Model file for the job. Use its own axes, mm. Coordinates: 2 decimals unless noted, no trailing zeros. Write each loop counter-clockwise with the first axis right and the second up, starting at its lowest first coordinate (ties: lowest second). Pieces come first, ordered by that corner, then holes. Notation, with made-up numbers: (-31.75, 86) - (-8.75, 86) arc R23 cw to (-8.75, 121) - close; hole circle Ø8 at (3.5, 52). An arc over 180 degrees is marked (long way). Put each result on its own line as item: value. Start each with the question number.
1. Drill centre lines: L1, parallel to Z at x = 47, y = -0.35; L2, parallel to Z at x = 45, y = -0.75; L3, parallel to Z at x = -49, y = -0.1. Where is each one in solid material? Low to high. Write a range as from..to.
2. Drop flat-ended pins along their axis: P1, Ø0.5, axis at y = -0.5, z = -14, coming from the -X side; P2, Ø5, axis at x = 40, z = -2.5, coming from the -Y side; P3, Ø0.5, axis at y = -0.5, z = -10.5, coming from the +X side. Give the stop position or say it passes through.
3. Saw through at A-A, the plane x = -18.5. Write the cut outline in (y, z), plus the area to 3 significant figures.
4. Saw through at C-C, the plane x = 20. Write the cut outline in (y, z).
5. Saw through at B-B, the plane y = -0.75. Give the number of separate pieces and of enclosed holes in the cut face, plus the area to 3 significant figures.
```python
from build123d import *

# Parameters (mm, degrees)
F0_W     = 0.1
F0_H     = 0.5
F0_W_2   = 4.5762195215
F0_H_2   = 0.1
F0_W_3   = 15
F0_H_3   = 7
F0_W_4   = 4
F0_W_5   = 5.7000000263
F0_W_6   = 6
F0_H_4   = 8
F0_W_7   = 2.1349615479
F0_W_8   = 5.4599995956
F0_H_5   = 1.8540623203
F0_H_6   = 1.1455476638
F0_W_9   = 7.5237791166
F0_W_10  = 2
F0_W_11  = 3.1167556109
F0_H_7   = 0.894062461
F0_W_12  = 8
F0_W_13  = 1.8985043958
F0_W_14  = 5.535091728
F0_W_15  = 2.1720023397
F0_W_16  = 5
F0_H_8   = 5
F0_W_17  = 9
F0_H_9   = 6
F0_W_18  = 3.3521689058
F1_DEPTH = 1


with BuildPart() as f1:
    # F0 (on Front) → F1 (new body)
    with BuildSketch(Plane.XZ):
        Polygon((-0.7164276307, -4), (-1.7164276307, -4), (-1.7164276307, 2.0474093835), (21.9873721178, 2.0474093835), (21.9873721178, -2.9525906165), (1.9873721178, -2.9525906165), (0.2835723693, -4), (-0.6164276307, -4), (-0.6164276307, -4.5), (0.4249689693, -4.5), (2.1287687179, -3.4525906165), (22.4873721178, -3.4525906165), (22.4873721178, -0.1), (22.4873721178, 0), (22.4873721178, 2.5474093835), (-2.2164276307, 2.5474093835), (-2.2164276307, 0), (-2.2164276307, -0.1), (-2.2164276307, -4.5), (-0.7164276307, -4.5), align=None)
        with Locations((-0.6664276307, -4.25)):
            Rectangle(F0_W, F0_H)
        with BuildLine():
            Line((-0.6164276307, -4.5), (-0.7164276307, -4.5))
            Line((-0.7164276307, -4.5), (-0.7164276307, -13.3747674979))
            ThreePointArc((-0.7164276307, -13.3747674979), (-0.6663757902, -13.3759068091), (-0.6164276307, -13.3793223828))
            Line((-0.6164276307, -13.3793223828), (-0.6164276307, -4.5))
        make_face()
        with BuildLine():
            ThreePointArc((-0.6164276307, -13.3793223828), (-0.6663757902, -13.3759068091), (-0.7164276307, -13.3747674979))
            ThreePointArc((-0.7164276307, -13.3747674979), (-1.8164276307, -14.4747674979), (-0.7164276307, -15.5747674979))
            Line((-0.7164276307, -15.5747674979), (-0.7164276307, -15.4747674979))
            ThreePointArc((-0.7164276307, -15.4747674979), (-1.4235344119, -13.7676607167), (0.2835723693, -14.4747674979))
            ThreePointArc((0.2835723693, -14.4747674979), (0.025192218, -15.1455878911), (-0.6164276307, -15.469754935))
            Line((-0.6164276307, -15.469754935), (-0.6164276307, -15.5702126129))
            ThreePointArc((-0.6164276307, -15.5702126129), (0.0559267082, -15.2580099731), (0.3775103589, -14.5900917138))
            ThreePointArc((0.3775103589, -14.5900917138), (0.3816245836, -14.5401994065), (0.3834645069, -14.4901715758))
            ThreePointArc((0.3834645069, -14.4901715758), (0.3835454033, -14.4824697256), (0.3835723693, -14.4747674979))
            ThreePointArc((0.3835723693, -14.4747674979), (0.0959762097, -13.7331476491), (-0.6164276307, -13.3793223828))
        make_face()
        with BuildLine():
            Line((-0.7164276307, -15.4747674979), (-0.7164276307, -15.5747674979))
            ThreePointArc((-0.7164276307, -15.5747674979), (-0.6663757902, -15.5736281866), (-0.6164276307, -15.5702126129))
            Line((-0.6164276307, -15.5702126129), (-0.6164276307, -15.469754935))
            ThreePointArc((-0.6164276307, -15.469754935), (-0.6663648557, -15.473513571), (-0.7164276307, -15.4747674979))
        make_face()
        with BuildLine():
            ThreePointArc((-0.6164276307, -15.5702126129), (-0.6663757902, -15.5736281866), (-0.7164276307, -15.5747674979))
            Line((-0.7164276307, -15.5747674979), (-0.7164276307, -16.196783632))
            Line((-0.7164276307, -16.196783632), (-0.6164276307, -16.196783632))
            Line((-0.6164276307, -16.196783632), (-0.6164276307, -15.5702126129))
        make_face()
        with Locations((-4.5045373915, -0.05)):
            Rectangle(F0_W_2, F0_H_2)
        Polygon((-6.7926471522, -5.3350963127), (-6.7926471522, -0.1), (-6.7926471522, 0), (-6.7926471522, 2.6649036873), (-22.7926471522, 2.6649036873), (-22.7926471522, 0), (-22.7926471522, -0.1), (-22.7926471522, -5.3350963127), align=None)
        with Locations((-14.7926471522, -1.3350963127)):
            Rectangle(F0_W_3, F0_H_3, mode=Mode.SUBTRACT)
        with BuildLine():
            Line((44.9668482701, -15.1770115764), (0.3834645069, -14.4901715758))
            ThreePointArc((0.3834645069, -14.4901715758), (0.3816245836, -14.5401994065), (0.3775103589, -14.5900917138))
            Line((0.3775103589, -14.5900917138), (44.9668482701, -15.2770234426))
            Line((44.9668482701, -15.2770234426), (45.0668482701, -15.2785640165))
            Line((45.0668482701, -15.2785640165), (45.0668482701, -15.1785521504))
            Line((45.0668482701, -15.1785521504), (45.0668482701, -13.2785640165))
            Line((45.0668482701, -13.2785640165), (44.9668482701, -13.2785640165))
            Line((44.9668482701, -13.2785640165), (44.9668482701, -15.1770115764))
        make_face()
        with Locations((24.4873721178, -0.05)):
            Rectangle(F0_W_4, F0_H_2)
        Polygon((26.4873721178, 0), (26.4873721178, -0.1), (26.4873721178, -2.6669805495), (29.4873721178, -3.0982994409), (29.5873721178, -3.1126767373), (32.4873721178, -3.5296183324), (32.4873721178, 0), (32.4873721178, 0.1), (32.4873721178, 2.5474093835), (26.4873721178, 2.5474093835), (26.4873721178, 0.0474093835), align=None)
        Polygon((26.9873721178, -2.2337257974), (26.9873721178, 0.0474093835), (26.9873721178, 2.0474093835), (31.9873721178, 2.0474093835), (31.9873721178, -2.9525906165), (29.5873721178, -2.6075355033), align=None, mode=Mode.SUBTRACT)
        Polygon((44.0542930675, -13.2785640165), (44.9668482701, -13.2785640165), (45.0668482701, -13.2785640165), (46.0794034727, -13.2785640165), (46.5562570157, -12.0984218523), (52.1539116397, -12.0984218523), (52.1539116397, -9.4984218523), (44.0542930675, -9.4984218523), (44.0542930675, -10.1705333218), (44.0542930675, -10.2705333218), align=None)
        Polygon((51.8539116397, -11.7984218523), (46.3539116397, -11.7984218523), (45.8770580967, -12.9785640165), (44.3542930675, -12.9785640165), (44.3542930675, -9.7984218523), (51.8539116397, -9.7984218523), align=None, mode=Mode.SUBTRACT)
        with Locations((-25.6426471653, -0.05)):
            Rectangle(F0_W_5, F0_H_2)
        Polygon((-28.4926471785, -6.3350963127), (-28.4926471785, -0.1), (-28.4926471785, 0), (-28.4926471785, 2.6649036873), (-35.4926471785, 2.6649036873), (-35.4926471785, 0), (-35.4926471785, -0.1), (-35.4926471785, -6.3350963127), align=None)
        with Locations((-31.9926471785, -1.8350963127)):
            Rectangle(F0_W_6, F0_H_4, mode=Mode.SUBTRACT)
        Polygon((29.5873721178, -3.1126767373), (29.4873721178, -3.0982994409), (29.4873721178, -8.2004475985), (32.0807600558, -8.2004475985), (32.1807600558, -8.2004475985), (36.7373721178, -8.2004475985), (36.7373721178, -1.7004475985), (36.6373721178, -1.7004475985), (36.6373721178, -8.1004475985), (29.5873721178, -8.1004475985), align=None)
        with Locations((42.9868122936, -10.2205333218)):
            Rectangle(F0_W_7, F0_H_2)
        Polygon((41.9193315196, -11.5084912181), (41.9193315196, -10.2705333218), (41.9193315196, -10.1705333218), (41.9193315196, -9.0544288978), (35.859331924, -9.0544288978), (35.859331924, -10.0930264927), (35.859331924, -10.1930264927), (35.859331924, -11.5084912181), align=None)
        with Locations((38.8893317218, -10.2814600579)):
            Rectangle(F0_W_8, F0_H_5, mode=Mode.SUBTRACT)
        with Locations((32.1307600558, -8.7732214304)):
            Rectangle(F0_W, F0_H_6)
        with Locations((-39.2545367368, -0.05)):
            Rectangle(F0_W_9, F0_H_2)
        with Locations((33.4873721178, 0.05)):
            Rectangle(F0_W_10, F0_H_2)
        Polygon((32.1807600558, -9.3459952623), (32.0807600558, -9.3459952623), (30.2440719174, -9.3459952623), (30.2440719174, -10.8400577232), (33.9608275283, -10.8400577232), (33.9608275283, -10.1930264927), (33.9608275283, -10.0930264927), (33.9608275283, -9.3459952623), align=None)
        with Locations((32.1024497228, -10.0930264927)):
            Rectangle(F0_W_11, F0_H_7, mode=Mode.SUBTRACT)
        Polygon((-43.016426295, -6.0529528502), (-43.016426295, -0.1), (-43.016426295, 0), (-43.016426295, 2.9470471498), (-52.016426295, 2.9470471498), (-52.016426295, -0.0529528502), (-52.016426295, -0.1529528502), (-52.016426295, -6.0529528502), align=None)
        with Locations((-47.516426295, -1.5529528502)):
            Rectangle(F0_W_12, F0_H_4, mode=Mode.SUBTRACT)
        Polygon((34.4873721178, 3.6967870891), (34.4873721178, 0.1), (34.4873721178, 0), (34.4873721178, -1.7004475985), (36.6373721178, -1.7004475985), (36.7373721178, -1.7004475985), (38.9873721178, -1.7004475985), (38.9873721178, 0.3627240414), (38.9873721178, 0.4627240414), (38.9873721178, 3.6967870891), align=None)
        Polygon((34.9873721178, -1.2004475985), (34.9873721178, 0), (34.9873721178, 3.1967870891), (38.4873721178, 3.1967870891), (38.4873721178, -1.2004475985), align=None, mode=Mode.SUBTRACT)
        with Locations((34.9100797262, -10.1430264927)):
            Rectangle(F0_W_13, F0_H_2)
        with Locations((-54.783972159, -0.1029528502)):
            Rectangle(F0_W_14, F0_H_2)
        with Locations((40.0733732877, 0.4127240414)):
            Rectangle(F0_W_15, F0_H_2)
        Polygon((-57.551518023, -3.0529528502), (-57.551518023, -0.1529528502), (-57.551518023, -0.0529528502), (-57.551518023, 2.9470471498), (-63.551518023, 2.9470471498), (-63.551518023, 0.1), (-63.551518023, 0), (-63.551518023, -3.0529528502), align=None)
        with Locations((-60.551518023, -0.0529528502)):
            Rectangle(F0_W_16, F0_H_8, mode=Mode.SUBTRACT)
        Polygon((41.1593744576, 3.7098635044), (41.1593744576, 0.4627240414), (41.1593744576, 0.3627240414), (41.1593744576, -3.2901364956), (51.1593744576, -3.2901364956), (51.1593744576, 0.1098635044), (51.1593744576, 0.2098635044), (51.1593744576, 3.7098635044), align=None)
        with Locations((46.1593744576, 0.2098635044)):
            Rectangle(F0_W_17, F0_H_9, mode=Mode.SUBTRACT)
        with Locations((-66.051518023, 0.05)):
            Rectangle(F0_W_16, F0_H_2)
        with Locations((52.8354589105, 0.1598635044)):
            Rectangle(F0_W_18, F0_H_2)
    extrude(amount=F1_DEPTH)


solid = f1.part
```
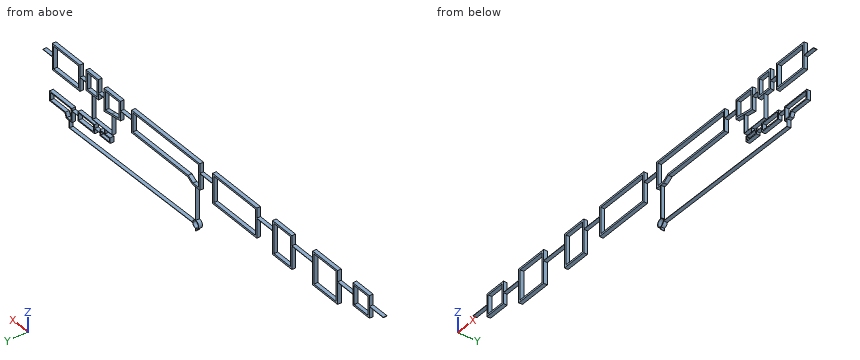
Final values:
1. L1: z = -12.1..-11.8, -9.8..-9.5, -3.29..-2.79, 3.21..3.71
1. L2: z = -15.28..-12.98, -9.8..-9.5, -3.29..-2.79, 3.21..3.71
1. L3: z = -6.05..-5.55, 2.45..2.95
2. P1: stops at x = -1.79
2. P2: stops at y = -1
2. P3: stops at x = 52.15
3. outline: (-1, -5.34) - (0, -5.34) - (0, -4.84) - (-1, -4.84) - close; (-1, 2.16) - (0, 2.16) - (0, 2.66) - (-1, 2.66) - close
3. area: 1.00 mm²
4. outline: (-1, -14.89) - (0, -14.89) - (0, -14.79) - (-1, -14.79) - close; (-1, -3.45) - (0, -3.45) - (0, -2.95) - (-1, -2.95) - close; (-1, 2.05) - (0, 2.05) - (0, 2.55) - (-1, 2.55) - close
5. separate pieces: 1
5. enclosed holes: 14
5. area: 159 mm²
